Geometry: final body of the model. Coordinates: model frame, mm. Give positions to 0.01 mm unless a question says otherwise; leave off trailing zeros. Write each loop counter-clockwise with the first axis right and the second up, starting at its lowest first coordinate (ties: lowest second). Pieces come first, ordered by that corner, then holes. Notation, with made-up numbers: (61.25, 69.25) -> (77.25, 69.25) arc R32 cw to (77.25, 105.25) -> close; hole circle Ø11 at (-14, 62.5). An arc over 180 degrees is marked (long way). Answer in a Markdown table with one row per item. Add a question column.
Item 1: First-contact query: P1, Ø4, axis at x = -181.92, z = 213.26, coming from the +Y side; P2, Ø0.8, axis at y = 1, z = 135, coming from the -X side; P3, Ø3, axis at x = -143.5, z = 137.65, coming from the -Y side. Flat tips, straight axial feed; report the tip coordinate or a pass-through.
Item 2: Section query B-B on z = 307. Output: boundary loops of the cut face in (x, y), plus the area to 3 significant figures.
Item 3: Section query A-A on y = 0.25. State how many separate pieces and enclosed holes the cut face has, plus the area to 3 significant figures.
Item 4: Section query C-C on x = -34. Output: boundary loops of the cut face in (y, z), plus the area to 3 significant figures.
Item 5: Material intervals for probe 1 along X at (y, z) = (1.4, 138); probe 2 along Z at (x, y) = (-98, 1.15); probe 3 along X at (y, z) = (1.4, 255.5), sorted ascending. Write a range as from..to.
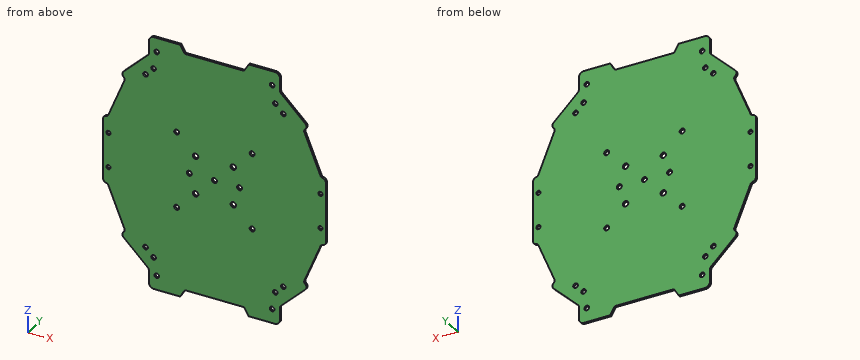
```python
from build123d import *

# Parameters (mm, degrees)
SKETCH1_R        = 2.2
SKETCH1_R_2      = 1.85915493
SKETCH1_R_3      = 2
SKETCH1_R_4      = 1.673239437
SKETCH1_R_5      = 1.983111479
EXTRUSION1_DEPTH = 1.6
FILLET1_R        = 1
FILLET2_R        = 4
FILLET3_R        = 3
FILLET4_R        = 3
FILLET5_R        = 2
FILLET6_R        = 2
FILLET7_R        = 3
FILLET8_R        = 3
FILLET9_R        = 2
FILLET10_R       = 2
FILLET11_R       = 3


with BuildPart() as part:
    # Sketch1 → Extrusion1 (new body)
    with BuildSketch(Plane(origin=(0, 0, 0), x_dir=(-1, 0, 0), z_dir=(0, 1, 0))):
        Polygon((74.087520418, 321.088295015), (70.369210559, 327.285477572), (45.580478165, 327.285477572), (45.580478165, 312.412238135), (23.246043749, 290.934342561), (26.682507041, 287.360833055), (12.735407819, 253.538985229), (9.017097883, 253.538985229), (9.017097883, 226.891111382), (9.017097883, 200.243237534), (12.735407819, 200.243237534), (26.682507041, 166.421389708), (23.246043749, 162.847880202), (45.580478165, 141.369984628), (45.580478165, 126.496745191), (70.369210559, 126.496745191), (74.087520418, 132.693927748), (97.636816193, 132.693927748), (121.186111968, 132.693927748), (124.904421827, 126.496745191), (149.693154221, 126.496745191), (149.693154221, 141.369984628), (172.027588636, 162.847880202), (168.591125345, 166.421389708), (182.538224567, 200.243237534), (186.256534503, 200.243237534), (186.256534503, 226.891111382), (186.256534503, 253.538985229), (182.538224567, 253.538985229), (168.591125345, 287.360833055), (172.027588636, 290.934342561), (149.693154221, 312.412238135), (149.693154221, 327.285477572), (124.904421827, 327.285477572), (121.186111968, 321.088295015), (97.636816193, 321.088295015), align=None)
        with Locations((112.636816193, 211.891111382)):
            Circle(SKETCH1_R, mode=Mode.SUBTRACT)
        with Locations((49.266182018, 151.62213525)):
            Circle(SKETCH1_R_2, mode=Mode.SUBTRACT)
        with Locations((112.636816193, 241.891111382)):
            Circle(SKETCH1_R, mode=Mode.SUBTRACT)
        with Locations((82.636816193, 241.891111382)):
            Circle(SKETCH1_R, mode=Mode.SUBTRACT)
        with Locations((82.636816193, 211.891111382)):
            Circle(SKETCH1_R, mode=Mode.SUBTRACT)
        with Locations((117.636816193, 226.891111382)):
            Circle(SKETCH1_R_3, mode=Mode.SUBTRACT)
        with Locations((77.636816193, 226.891111382)):
            Circle(SKETCH1_R_3, mode=Mode.SUBTRACT)
        with Locations((97.636816193, 226.891111382)):
            Circle(SKETCH1_R_3, mode=Mode.SUBTRACT)
        with Locations((51.777661187, 316.130534525)):
            Circle(SKETCH1_R_2, mode=Mode.SUBTRACT)
        with Locations((49.266182018, 302.160087513)):
            Circle(SKETCH1_R_2, mode=Mode.SUBTRACT)
        with Locations((13.355125975, 240.524915841)):
            Circle(SKETCH1_R_4, mode=Mode.SUBTRACT)
        with Locations((143.495971199, 137.651688238)):
            Circle(SKETCH1_R_2, mode=Mode.SUBTRACT)
        with Locations((146.007450368, 151.62213525)):
            Circle(SKETCH1_R_2, mode=Mode.SUBTRACT)
        with Locations((143.495971199, 316.130534525)):
            Circle(SKETCH1_R_2, mode=Mode.SUBTRACT)
        with Locations((181.918506411, 240.524915841)):
            Circle(SKETCH1_R_4, mode=Mode.SUBTRACT)
        with Locations((146.007450368, 302.160087513)):
            Circle(SKETCH1_R_2, mode=Mode.SUBTRACT)
        with Locations((181.918506411, 213.257306923)):
            Circle(SKETCH1_R_4, mode=Mode.SUBTRACT)
        with Locations((13.355125975, 213.257306923)):
            Circle(SKETCH1_R_4, mode=Mode.SUBTRACT)
        with Locations((51.777661187, 137.651688238)):
            Circle(SKETCH1_R_2, mode=Mode.SUBTRACT)
        with Locations((67.636816193, 196.891111382)):
            Circle(SKETCH1_R_5, mode=Mode.SUBTRACT)
        with Locations((67.636816193, 256.891111382)):
            Circle(SKETCH1_R_5, mode=Mode.SUBTRACT)
        with Locations((42.888078851, 158.000238416)):
            Circle(SKETCH1_R_2, mode=Mode.SUBTRACT)
        with Locations((152.385553534, 295.781984347)):
            Circle(SKETCH1_R_2, mode=Mode.SUBTRACT)
        with Locations((42.888078851, 295.781984347)):
            Circle(SKETCH1_R_2, mode=Mode.SUBTRACT)
        with Locations((127.636816193, 256.891111382)):
            Circle(SKETCH1_R_5, mode=Mode.SUBTRACT)
        with Locations((152.385553534, 158.000238416)):
            Circle(SKETCH1_R_2, mode=Mode.SUBTRACT)
        with Locations((127.636816193, 196.891111382)):
            Circle(SKETCH1_R_5, mode=Mode.SUBTRACT)
    extrude(amount=EXTRUSION1_DEPTH)

    # Fillet1
    fillet1_edges = [part.edges().sort_by_distance(p)[0] for p in [
        (-121.186111968, 0.8, 321.088295015),
        (-121.186111968, 0.8, 132.693927748),
        (-74.087520418, 0.8, 132.693927748),
        (-74.087520418, 0.8, 321.088295015),
    ]]
    fillet(fillet1_edges, radius=FILLET1_R)

    # Fillet2
    fillet2_edges = [part.edges().sort_by_distance(p)[0] for p in [
        (-149.693154221, 0.8, 327.285477572),
        (-149.693154221, 0.8, 126.496745191),
        (-45.580478165, 0.8, 126.496745191),
        (-45.580478165, 0.8, 327.285477572),
    ]]
    fillet(fillet2_edges, radius=FILLET2_R)

    # Fillet3
    fillet3_edges = [part.edges().sort_by_distance(p)[0] for p in [
        (-149.693154221, 0.8, 312.412238135),
        (-149.693154221, 0.8, 141.369984628),
        (-45.580478165, 0.8, 141.369984628),
        (-45.580478165, 0.8, 312.412238135),
    ]]
    fillet(fillet3_edges, radius=FILLET3_R)

    # Fillet4
    fillet4_edges = [part.edges().sort_by_distance(p)[0] for p in [
        (-172.027588636, 0.8, 290.934342561),
    ]]
    fillet(fillet4_edges, radius=FILLET4_R)

    # Fillet5
    fillet5_edges = [part.edges().sort_by_distance(p)[0] for p in [
        (-168.591125345, 0.8, 287.360833055),
    ]]
    fillet(fillet5_edges, radius=FILLET5_R)

    # Fillet6
    fillet6_edges = [part.edges().sort_by_distance(p)[0] for p in [
        (-26.682507041, 0.8, 287.360833055),
    ]]
    fillet(fillet6_edges, radius=FILLET6_R)

    # Fillet7
    fillet7_edges = [part.edges().sort_by_distance(p)[0] for p in [
        (-23.246043749, 0.8, 290.934342561),
    ]]
    fillet(fillet7_edges, radius=FILLET7_R)

    # Fillet8
    fillet8_edges = [part.edges().sort_by_distance(p)[0] for p in [
        (-172.027588636, 0.8, 162.847880202),
        (-23.246043749, 0.8, 162.847880202),
    ]]
    fillet(fillet8_edges, radius=FILLET8_R)

    # Fillet9
    fillet9_edges = [part.edges().sort_by_distance(p)[0] for p in [
        (-168.591125345, 0.8, 166.421389708),
        (-26.682507041, 0.8, 166.421389708),
    ]]
    fillet(fillet9_edges, radius=FILLET9_R)

    # Fillet10
    fillet10_edges = [part.edges().sort_by_distance(p)[0] for p in [
        (-182.538224567, 0.8, 253.538985229),
        (-182.538224567, 0.8, 200.243237534),
        (-12.735407819, 0.8, 200.243237534),
        (-12.735407819, 0.8, 253.538985229),
    ]]
    fillet(fillet10_edges, radius=FILLET10_R)

    # Fillet11
    fillet11_edges = [part.edges().sort_by_distance(p)[0] for p in [
        (-186.256534503, 0.8, 200.243237534),
        (-186.256534503, 0.8, 253.538985229),
        (-9.017097883, 0.8, 253.538985229),
        (-9.017097883, 0.8, 200.243237534),
    ]]
    fillet(fillet11_edges, radius=FILLET11_R)


solid = part.part
```
Findings below:
| question | item | result |
|---|---|---|
| 1 | P1 | stops at y = 1.6 |
| 1 | P2 | stops at x = -149.69 |
| 1 | P3 | passes through |
| 2 | outline | (-155.32, 0) -> (-39.95, 0) -> (-39.95, 1.6) -> (-155.32, 1.6) -> close |
| 2 | area | 185 mm^2 |
| 3 | separate pieces | 1 |
| 3 | enclosed holes | 27 |
| 3 | area | 28,600 mm^2 |
| 4 | outline | (0, 152.51) -> (1.6, 152.51) -> (1.6, 301.28) -> (0, 301.28) -> close |
| 4 | area | 238 mm^2 |
| 5 | probe 1 | x = -149.69..-145.32, -141.67..-53.6, -49.95..-45.58 |
| 5 | probe 2 | z = 132.69..224.92, 228.86..321.09 |
| 5 | probe 3 | x = -181.73..-129.05, -126.22..-69.05, -66.22..-13.54 |
